The model under review builds one solid part; all positions refer to its coordinate system, in mm. A direction names the side the tool comes from. Coordinates: 2 decimals unless noted, no trailing zeros. Order: outer loops, then holes, each group sorted by start corner. A loop starts at its lowest first (then second) coordinate and runs counter-clockwise, first axis right, second up. Notation, with made-up numbers: (49.25, 83) -> (90.25, 83) arc R17 cw to (90.25, 107) -> close; hole circle Ø5 at (60, 79.25). An arc over 180 degrees is marked (long way). Use CSV: the item, a comma, the result in double quotes. Start each with the question number.
```python
from build123d import *

# Parameters (mm, degrees)
F1_DEPTH = 9.525
F2_R     = 34.925
F3_DEPTH = 15.875
F4_R     = 19.05
F4_R_2   = 12.7
F5_DEPTH = 25.401
F6_R     = 0.79375


with BuildPart() as f1:
    # F0 (on Top) → F1 (new body)
    with BuildSketch(Plane.XY):
        with BuildLine():
            Line((122.766667, 75.728169), (9.877778, 88.34953))
            ThreePointArc((9.877778, 88.34953), (-88.9, 0), (9.877778, -88.34953))
            Line((9.877778, -88.34953), (122.766667, -75.728169))
            ThreePointArc((122.766667, -75.728169), (190.5, 0), (122.766667, 75.728169))
        make_face()
    extrude(amount=F1_DEPTH)

    # F2 (on face) → F3 (join)
    with BuildSketch(Plane.XY.offset(9.525)):
        Circle(F2_R)
    extrude(amount=F3_DEPTH)

    # F4 (on face) → F5 (cut, through all)
    with BuildSketch(Plane.XY.offset(25.4)):
        Circle(F4_R)
        with Locations((114.3, 0)):
            Circle(F4_R_2)
    extrude(amount=-F5_DEPTH, mode=Mode.SUBTRACT)

    # F6
    f6_edges = [f1.edges().sort_by_distance(p)[0] for p in [
        (-34.925, 0, 9.525),
        (-34.925, 0, 25.4),
        (190.5, 0, 9.525),
        (66.322222, -82.03885, 9.525),
        (-88.9, 0, 9.525),
        (66.322222, 82.03885, 9.525),
        (101.6, 0, 9.525),
    ]]
    fillet(f6_edges, radius=F6_R)


solid = f1.part
```
Q1. Draft analysis for pull direction Y (two halves, no side actions). For faces 1 (the flat face through (15, -15, 25.4)), 2 (the cylindrical face through (67.087, -81.726, 9.286)), 3 (the cylindrical face through (-15.12, -11.59, 12.88)), state which applies: +Y half, -Y half, draft (parallel to the pull), parting line (faces both ways), or undercut.
Q2. To check wall thickness, follow probe 1 along X at (y, z) = (5, 4.25); probe 2 along Z at (x, y) = (128, 52) (3 decimals); probe 3 along Y at (x, z) = (0, 12) (3 decimals). State the ranges of each line that lie inside material, in increasing order.
Q3. Add section B-B, the plane z = 5.5. State the section outline as (x, y) points, then the cut area to 3 significant figures.
Q4. Add section A-A, the plane y = 0. State how many separate pieces and enclosed holes the cut face has, then the cut area to 3 significant figures.
Q5. Clearance check with flat-ended pins moving along their axes: pin 1 Ø1 at (x, z) = (-15, 20.5) entering from +Y; pin 2 Ø3 at (y, z) = (6.5, 20.5) entering from -X; pin 3 Ø4 at (x, y) = (52, 37.5) entering from +Z (3 decimals). State where each tip first meets the part, or that it passes through.
Q6. For faces 4 (the cylindrical face through (-27.715, -21.251, 17.362)), 5 (the cylindrical face through (65.51, 81.9, 9.29)), list the 3-axis set-ups (+Z, -Z, +X, -X, +Y, -Y) from which the entire face can be reached by the end or side of a thin tool; tool diameter is ignored.
Answer block:
1,face 1,"draft"
1,face 2,"-Y half"
1,face 3,"undercut"
2,probe 1,"x = -88.76 to -18.38, 18.38 to 102.63, 125.97 to 190.34"
2,probe 2,"z = 0 to 9.525"
2,probe 3,"y = -34.925 to -19.05, 19.05 to 34.925"
3,outline,"(9.88, -88.35) -> (122.77, -75.73) arc R76.2 ccw to (122.77, 75.73) -> (9.88, 88.35) arc R88.9 ccw (long way) to start; hole circle Ø38.1 at (0, 0); hole circle Ø25.4 at (114.3, 0)"
3,area,"38,900 mm²"
4,separate pieces,"3"
4,enclosed holes,"0"
4,area,"2,560 mm²"
5,pin 1,"stops at y = 31.77"
5,pin 2,"stops at x = -34.57"
5,pin 3,"stops at z = 9.525"
6,face 4,"+Z"
6,face 5,"+Z, +X, +Y"
